Design review of the part built by this model. Coordinates are the model's own, in mm. A direction names the side the tool comes from. Round coordinates to 2 decimals unless told otherwise and drop trailing zeros. Loops run counter-clockwise (first coordinate to the right, second up) from the corner with the lowest first, then second, coordinate; pieces in that order, holes last. Notation, with made-up numbers: (29.25, 33.5) - (35.25, 33.5) arc R31 cw to (35.25, 72.5) - close; hole circle Ø9 at (17, 13.5). An arc over 180 degrees is marked (long way). Return JSON: item names as keys, results as strings. Group by question number.
(1) We need section C-C, the plane y = 45. Write out the cut boundary in (x, z).
(2) We need section D-D, the plane x = 61.5. Write out the cut boundary in (y, z).
(3) Clearance check with flat-ended pins moving along their axes: pin 1 (6 mm diameter, centred on x = 94, z = 27.5, fed in from -Y); pin 2 (10 mm diameter, centred on y = -7, z = 40.5, fed in from -X); pin 3 (4 mm diameter, centred on x = 60.5, z = 7.5, fed in from -Y). State where each tip first meets the part, or that it passes through.
(4) For faces 5 (the flat face through (70, 13, 0)), 6 (the flat face through (12, 25, 50)), 7 (the flat face through (21, 0, 4)), 8 (the flat face through (59, 50, 4)), 9 (the flat face through (90, 30, 37)), list the 3-axis set-ups (+Z, -Z, +X, -X, +Y, -Y) from which the entire face can be reached by the end or side of a thin tool; tool diameter is ignored.
(5) We need section A-A, the plane z = 42.5. Write out the cut boundary in (x, y), and give its area (3 significant figures).
(6) We need section B-B, the plane y = 3. Write out the cut boundary in (x, z), and give its area (3 significant figures).
(7) Wall thickness on L1, parallel to X at y = 38, z = 32; L2, parallel to Y at x = 54.5, z = 21.5; L3, parallel to Z at x = 72, y = 39.5: over which ranges is each line inside the solid? List them lowest first. Write a range as [from, to].
(8) The part is to be moulded in two halves that separate along X. For faces 1 (the flat face through (108, 15, 50)), 2 (the flat face through (57, 31, 25)), 3 (the flat face through (0, 25, 12)), 4 (the flat face through (120, 15, 13)), say which applies: pulls with the +X half, pulls with the -X half, needs draft (parallel to the pull), parting line crosses it, or undercut.
from build123d import *

# Parameters (mm, degrees)
F0_W     = 25
F0_H     = 50
F1_DEPTH = 25
F2_W     = 25
F2_H     = 50
F3_DEPTH = 25


with BuildPart() as f1:
    # F0 (on Top) → F1 (new body, symmetric)
    with BuildSketch(Plane.XY):
        with Locations((12.5, 25)):
            Rectangle(F0_W, F0_H)
        Polygon((25, 50), (25, 0), (42.5, 0), (42.5, 15), (70, 15), (70, 10), (100, 10), (100, -20), (120, -20), (120, 50), align=None)
    extrude(amount=F1_DEPTH, both=True)

    # F2 (on face) → F3 (join)
    with BuildSketch(Plane.XY.offset(25)):
        with Locations((12.5, 25)):
            Rectangle(F2_W, F2_H)
        Polygon((100, -20), (120, -20), (120, 50), (90, 50), (90, 10), (100, 10), align=None)
    extrude(amount=F3_DEPTH)


solid = f1.part
Solutions:
{
 "1": {"outline": "(0, -25) - (120, -25) - (120, 50) - (90, 50) - (90, 25) - (25, 25) - (25, 50) - (0, 50) - close"},
 "2": {"outline": "(15, -25) - (50, -25) - (50, 25) - (15, 25) - close"},
 "3": {"pin 1": "y = 10", "pin 2": "x = 100", "pin 3": "y = 15"},
 "4": {"face 5": "+Z, -Z, -Y", "face 6": "+Z, +X, -X, +Y, -Y", "face 7": "+Z, -Z, -X, -Y", "face 8": "+Z, -Z, +X, -X, +Y", "face 9": "+Z, +Y, -Y"},
 "5": {"outline": "(0, 0) - (25, 0) - (25, 50) - (0, 50) - close; (90, 10) - (100, 10) - (100, -20) - (120, -20) - (120, 50) - (90, 50) - close", "area": "3,050 mm^2"},
 "6": {"outline": "(0, -25) - (42.5, -25) - (42.5, 25) - (25, 25) - (25, 50) - (0, 50) - close; (100, -25) - (120, -25) - (120, 50) - (100, 50) - close", "area": "4,250 mm^2"},
 "7": {"L1": "[0, 25], [90, 120]", "L2": "[15, 50]", "L3": "[-25, 25]"},
 "8": {"face 1": "needs draft", "face 2": "undercut", "face 3": "pulls with the -X half", "face 4": "pulls with the +X half"}
}
